Check sheet for the modelled part. Datum: model origin and axes. Units: mm. A direction names the side the tool comes from. Give positions to 0.01 mm unless a question says otherwise; leave off trailing zeros. Write item = value, one per line. Start each with the question number.
1) Set-up check for faces 1 (the face through (100, 2, 5)), 2 (the face through (110, 0, 5)), 3 (the face through (-106, -2.5, 2.4)): record each of +Z, -Z, +X, -X, +Y, -Y from which the full face is reachable in a straight line by a thin tool's end or side.
2) Sectioned sample at A-A, the plane y = 0. Count the separate pieces of the cut face and the enclosed holes in it, then the cut area to 3 significant figures.
3) Scan lines: L1, parallel to X at y = 0, z = 8.05 (3 decimals); L2, parallel to X at y = -1.5, z = 9; L3, parallel to Y at x = -100, z = 5.75 (3 decimals). Record each from-to range of solid material in increasing order.
4) Gauge pin test, flat ends, axial feed: pin 1 (4 mm diameter, centred on x = -100, y = 0, fed in from -Z); pin 2 (8 mm diameter, centred on x = -100, y = 0, fed in from -Z); pin 3 (6.5 mm diameter, centred on x = -98, y = -3, fed in from -Z); pin 4 (1 mm diameter, centred on y = -4.5, z = 1.5, fed in from +X). Record the tip position at first contact, or that the pin passes through.
from build123d import *

# Parameters (mm, degrees)
SKETCH1_R           = 2.625
BOSS_EXTRUDE1_DEPTH = 10
SKETCH2_R           = 6.5
CUT_EXTRUDE1_DEPTH  = 4
CHAMFER1_SIZE       = 0.75


with BuildPart() as part:
    # Sketch1 → Boss-Extrude1 (new body)
    with BuildSketch(Plane.XY):
        with BuildLine():
            Line((100, 10), (-100, 10))
            ThreePointArc((-100, 10), (-110, 0), (-100, -10))
            Line((-100, -10), (100, -10))
            ThreePointArc((100, -10), (110, 0), (100, 10))
        make_face()
        with Locations((-100, 0)):
            Circle(SKETCH1_R, mode=Mode.SUBTRACT)
        with BuildLine():
            Line((98.338675227, 2), (101.661324773, 2))
            ThreePointArc((101.661324773, 2), (100, -2.6), (98.338675227, 2))
        make_face(mode=Mode.SUBTRACT)
    extrude(amount=BOSS_EXTRUDE1_DEPTH)

    # Sketch2 → Cut-Extrude1 (cut)
    with BuildSketch(Plane(origin=(0, 0, 0), x_dir=(-1, 0, 0), z_dir=(0, 0, -1))):
        with Locations((100, 0)):
            Circle(SKETCH2_R)
    extrude(amount=-CUT_EXTRUDE1_DEPTH, mode=Mode.SUBTRACT)

    # Chamfer1
    chamfer1_edges = [part.edges().sort_by_distance(p)[0] for p in [
        (-110, 0, 0),
        (0, 10, 0),
        (110, 0, 0),
        (110, 0, 10),
        (0, -10, 0),
        (0, 10, 10),
        (-110, 0, 10),
        (-102.625, 0, 4),
        (-93.5, 0, 0),
        (-102.625, 0, 10),
        (100, -2.6, 10),
        (100, 2, 10),
        (0, -10, 10),
        (100, 2, 0),
        (100, -2.6, 0),
    ]]
    chamfer(chamfer1_edges, length=CHAMFER1_SIZE)


solid = part.part
Data:
q1.face_1 = +Z, -Z
q1.face_2 = +Z, -Z, +X
q1.face_3 = -Z
q2.separate_pieces = 3
q2.enclosed_holes = 0
q2.area = 2,060 mm2
q3.L1 = -110 to -102.625, -97.375 to 97.4, 102.6 to 110
q3.L2 = -109.89 to -102.15, -97.85 to 97.88, 102.12 to 109.89
q3.L3 = -10 to -2.625, 2.625 to 10
q4.pin_1 = through
q4.pin_2 = 4
q4.pin_3 = 0.39
q4.pin_4 = 109.17
